The listing builds one solid part. Answer for the finished solid, in the listing's coordinates (mm). Give positions to 0.01 mm unless a question says otherwise; leave off trailing zeros. Order: outer loops, then holes, each group sorted by start corner. A loop starts at its lowest first (then second) coordinate and runs counter-clockwise, first axis right, second up. Notation, with made-up numbers: (15.25, 1) - (19.25, 1) arc R24 cw to (19.25, 36) - close; hole circle Ø10 at (51, 86). An arc over 180 degrees is marked (long way). Write each question's results on one line, items separated by ' | '. Start each with the question number.
1. Section B-B (x = -145) is taken. Give the vertices of the cut face in (y, z).
2. Flat-ended cylindrical pins translate along their axes: pin 1 (3 mm diameter, centred on y = 0.5, z = -57, fed in from +X); pin 2 (2 mm diameter, centred on x = 201, y = 1.5, fed in from +Z); pin 3 (1 mm diameter, centred on x = 161.5, y = 3.5, fed in from -Z). Find the tip coordinate at first contact, or state that the pin passes through.
3. Find the intervals of material crossed by L1, parallel to Z at x = -8.5, y = 5.2; L2, parallel to X at y = 0.4, z = -252; L3, parallel to X at y = 4.8, z = 225.5, in increasing order.
4. Section C-C (x = 56) is taken. Give the vertices of the cut face in (y, z), and give its area (3 significant figures).
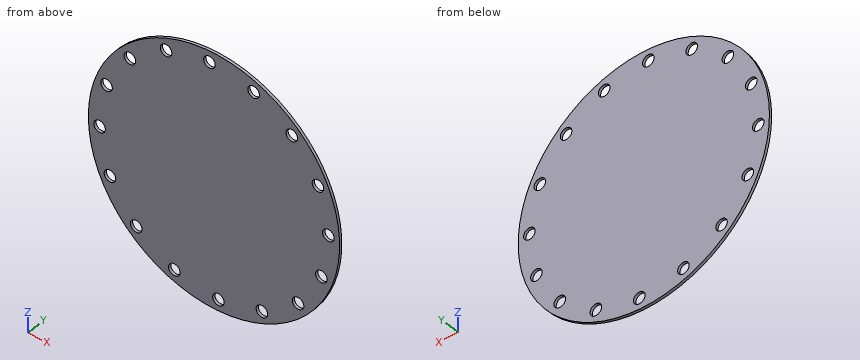
Autodesk Inventor part; units mm, degrees
ref_plane "YZ Plane" through (0, 0, 0) normal (1, 0, 0) x (0, 1, 0)
ref_plane "XZ Plane" through (0, 0, 0) normal (0, 1, 0) x (-1, 0, 0)
ref_plane "XY Plane" through (0, 0, 0) normal (0, 0, 1) x (1, 0, 0)
sketch "Sketch1" plane through (0, 0, 0) normal (0, 1, 0) x (-1, 0, 0)
  circle A0 centre (0, 0) radius 282.5
  dimension "d0" = 565
extrude "Extrusion1" add sketch "Sketch1" along normal blind 6
sketch "Sketch2" plane through (0, 6, 0) normal (0, 1, 0) x (1, 0, 0)
  circle A0 centre (0, 0) radius 257.5 construction
  line L0 (0, 0) -> (-257.5, 0)
  line L1 (0, 0) -> (-241.5843, -89.1251) construction
  circle A1 centre (-241.5843, -89.1251) radius 13
  dimension "d4" = 515
  dimension "d15" = 20.25
  dimension "d16" = 26
extrude "Cut1" cut sketch "Sketch2" against normal through all
pattern_circular "Circular Pattern1" count 16 over 360 about axis through (0, 0, 0) along (0, 1, 0) of "Cut1"
equation "\"d6\" = Thickness"
equation "\"BendRadius\" = Thickness"
equation "\"BendReliefWidth\" = Thickness"
equation "\"BendReliefDepth\" = 0.5 * Thickness"
equation "\"CornerReliefSize\" = 4 * Thickness"
equation "\"MinimumRemnant\" = 2 * Thickness"
equation "\"TransitionRadius\" = BendRadius"
equation "\"JacobiRadiusSize\" = BendRadius"
equation "\"GapSize\" = Thickness"
equation "\"d5\" = Thickness"
properties part number "TZS 1212 charging hatch 500 mm" material "Steel"
Reported:
1) outline: (0, -242.45) - (6, -242.45) - (6, 242.45) - (0, 242.45) - close
2) pin 1: x = 276.99 | pin 2: z = 199.52 | pin 3: z = -232.13
3) L1: -282.37 to 244.4, 270.2 to 282.37 | L2: -127.68 to -96.9, -81.35 to -1.76, 21.98 to 127.68 | L3: -170.16 to -117.77, -97.84 to 170.16
4) outline: (0, -276.89) - (6, -276.89) - (6, 276.89) - (0, 276.89) - close | area: 3,320 mm²
